```python
from build123d import *

# Parameters (mm, degrees)
F0_W     = 50.8
F0_H     = 50.8
F0_R     = 9.781651
F1_DEPTH = 50.8
F2_W     = 18.904511
F2_H     = 19.477375
F3_DEPTH = 8.636
F4_DEPTH = 8.89
F5_R     = 10.389056
F6_DEPTH = 11.176


with BuildPart() as f1:
    # F0 (on Front) → F1 (new body)
    with BuildSketch(Plane.XZ):
        with Locations((-25.4, 25.4)):
            Rectangle(F0_W, F0_H)
        with Locations((-25.969833, 23.869332)):
            Circle(F0_R, mode=Mode.SUBTRACT)
    extrude(amount=F1_DEPTH)

    # F2 (on face) → F3 (join)
    with BuildSketch(Plane.YZ):
        with Locations((-26.638174, 28.452244)):
            Rectangle(F2_W, F2_H)
    extrude(amount=F3_DEPTH)

    # F2 (on face) → F4 (join)
    with BuildSketch(Plane.YZ):
        with Locations((-26.638174, 28.452244)):
            Rectangle(F2_W, F2_H)
    extrude(amount=F4_DEPTH)

    # F5 (on face) → F6 (join)
    with BuildSketch(Plane(origin=(0, 0, 0), x_dir=(1, 0, 0), z_dir=(0, 0, -1))):
        with Locations((-25.969833, 25.01506)):
            Circle(F5_R)
    extrude(amount=F6_DEPTH)


solid = f1.part
```
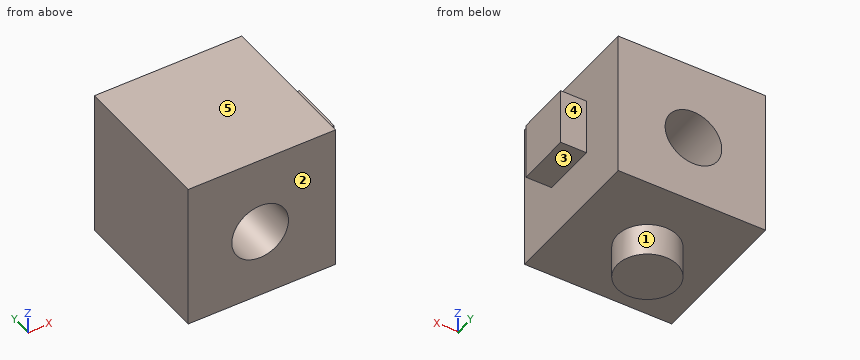
Could you check a few things on this model? Use its own coordinates, in mm. Face numbers are marked on the shaded views. A direction names the side the tool comes from. Coordinates: 2 decimals unless noted, no trailing zeros. Loops run counter-clockwise (first coordinate to the right, second up) from the corner with the lowest first, then second, coordinate; pieces in that order, holes last.
1) Imagine slicing it at D-D (z = 40.5). List the corners of the cut face in (x, y) for me, and give its area (3 significant figures).
Reported:
outline: (-50.8, -50.8) - (0, -50.8) - (0, 0) - (-50.8, 0) - close
area: 2,580 mm2
2) Imagine slicing it at B-B (z = 23). List the corners of the cut face in (x, y) for me, and give its area (3 significant figures).
Reported:
outline: (-50.8, -50.8) - (-35.71, -50.8) - (-35.71, 0) - (-50.8, 0) - close; (-16.23, -50.8) - (0, -50.8) - (0, -36.09) - (8.89, -36.09) - (8.89, -17.19) - (0, -17.19) - (0, 0) - (-16.23, 0) - close
area: 1,760 mm2
3) Imagine slicing it at A-A (x = -24). List the corners of the cut face in (y, z) for me.
Reported:
outline: (-50.8, 0) - (-35.22, 0) - (-35.22, -11.18) - (-14.81, -11.18) - (-14.81, 0) - (0, 0) - (0, 14.29) - (-50.8, 14.29) - close; (-50.8, 33.45) - (0, 33.45) - (0, 50.8) - (-50.8, 50.8) - close
4) Please list where these lines run through material, in increasing order: line 1 along X through (y, z) = (-33.5, 12.5); line 2 along Z through (x, y) = (-26, -36.5); line 3 along X through (y, z) = (-21, 19).
Reported:
line 1: x = -50.8 to 0
line 2: z = 0 to 14.09, 33.65 to 50.8
line 3: x = -50.8 to -34.45, -17.49 to 8.89
5) Will these pins go through, and if not, where does the flat tip stop? pin 1 Ø1 at (x, z) = (1.5, 28.5) entering from -Y; pin 2 Ø4 at (y, z) = (-12, 31.5) entering from +X; pin 3 Ø7 at (x, y) = (4.5, -28.5) entering from +Z.
Reported:
pin 1: stops at y = -36.09
pin 2: stops at x = 0
pin 3: stops at z = 38.19
6) Imagine slicing it at C-C (y = -21.5). List the corners of the cut face in (x, z) for me.
Reported:
outline: (-50.8, 0) - (-35.75, 0) - (-35.75, -11.18) - (-16.19, -11.18) - (-16.19, 0) - (0, 0) - (0, 18.71) - (8.89, 18.71) - (8.89, 38.19) - (0, 38.19) - (0, 50.8) - (-50.8, 50.8) - close; hole circle Ø19.56 at (-25.97, 23.87)
7) Which directions (+Z, -Z, +X, -X, +Y, -Y) give clear straight access to the entire face, cutting with the end or side of a thin tool? Please do the marked faces 1, 2, 3, 4 and 5.
Reported:
face 1: -Z
face 2: +Z, -Z, +X, -X, -Y
face 3: -Z, +X, +Y, -Y
face 4: +Z, -Z, +X, +Y
face 5: +Z, +X, -X, +Y, -Y
